Source: CAD feature listing. Evaluate the final solid. Frame: model axes, mm. Face numbers are marked on the shaded views. A direction names the side the tool comes from. Give positions to 0.01 mm unless a question says otherwise; leave off trailing zeros. Loops run counter-clockwise (first coordinate to the right, second up) from the corner with the lowest first, then second, coordinate; pieces in that order, holes last.
from build123d import *

# Parameters (mm, degrees)
SKETCH1_R           = 16
BOSS_EXTRUDE1_DEPTH = 850
SKETCH2_R           = 14.5
CUT_EXTRUDE1_DEPTH  = 848
BOSS_EXTRUDE2_START = -2
SKETCH3_R           = 17
SKETCH3_R_2         = 16
BOSS_EXTRUDE2_DEPTH = 2
FILLET1_R           = 1.5
SKETCH4_R           = 17
SKETCH4_R_2         = 16
BOSS_EXTRUDE3_DEPTH = 2
FILLET2_R           = 1.5


with BuildPart() as part:
    # Sketch1 → Boss-Extrude1 (new body)
    with BuildSketch(Plane(origin=(0, 0, 0), x_dir=(1, 0, 0), z_dir=(0, 1, 0))):
        with Locations(Location((0, 0, 0), (0, 0, 270))):
            Circle(SKETCH1_R)
    extrude(amount=BOSS_EXTRUDE1_DEPTH)

    # Sketch2 → Cut-Extrude1 (cut)
    with BuildSketch(Plane(origin=(0, 850, 0), x_dir=(1, 0, 0), z_dir=(0, 1, 0))):
        with Locations(Location((0, 0, 0), (0, 0, 270))):
            Circle(SKETCH2_R)
    extrude(amount=-CUT_EXTRUDE1_DEPTH, mode=Mode.SUBTRACT)

    # Sketch3 → Boss-Extrude2 (add)
    with BuildSketch(Plane(origin=(0, 800, 0), x_dir=(1, 0, 0), z_dir=(0, 1, 0)).offset(BOSS_EXTRUDE2_START)):
        with Locations(Location((0, 0, 0), (0, 0, 270))):
            Circle(SKETCH3_R)
        with Locations(Location((0, 0, 0), (0, 0, 270))):
            Circle(SKETCH3_R_2, mode=Mode.SUBTRACT)
    extrude(amount=BOSS_EXTRUDE2_DEPTH)

    # Fillet1
    # the kernel refuses this fillet: 1.5 mm, written as the material it takes off along each edge
    with BuildSketch(Plane(origin=(0, 798, 0), x_dir=(0, 0, 1), z_dir=(-1, 0, 0))) as fillet1_piece_1:
        with BuildLine():
            CenterArc((15.5, 1.414213562), FILLET1_R, 289.471220634, 70.528779366)
            Line((17, 1.414213562), (17.03, 1.414213562))
            Line((17.03, 1.414213562), (17.03, 0))
            Line((17.03, 0), (17, -0.03))
            ThreePointArc((17, -0.03), (16.5, -0.03), (16.01, -0.028284271))
            Line((16.01, -0.028284271), (16, 0))
        make_face()
    revolve(axis=Axis((0, 798, 0), (0, 1, 0)), mode=Mode.SUBTRACT)

    # Sketch4 → Boss-Extrude3 (add)
    with BuildSketch(Plane(origin=(0, 640, 0), x_dir=(1, 0, 0), z_dir=(0, 1, 0))):
        with Locations(Location((0, 0, 0), (0, 0, 270))):
            Circle(SKETCH4_R)
        with Locations(Location((0, 0, 0), (0, 0, 270))):
            Circle(SKETCH4_R_2, mode=Mode.SUBTRACT)
    extrude(amount=BOSS_EXTRUDE3_DEPTH)

    # Fillet2
    # the kernel refuses this fillet: 1.5 mm, written as the material it takes off along each edge
    with BuildSketch(Plane(origin=(0, 642, 0), x_dir=(0, 0, 1), z_dir=(-1, 0, 0))) as fillet2_piece_1:
        with BuildLine():
            CenterArc((15.5, -1.414213562), FILLET2_R, 0, 70.528779366)
            Line((16, 0), (16.01, 0.028284271))
            ThreePointArc((16.01, 0.028284271), (16.5, 0.03), (17, 0.03))
            Line((17, 0.03), (17.03, 0))
            Line((17.03, 0), (17.03, -1.414213562))
            Line((17.03, -1.414213562), (17, -1.414213562))
        make_face()
    revolve(axis=Axis((0, 642, 0), (0, 1, 0)), mode=Mode.SUBTRACT)


solid = part.part
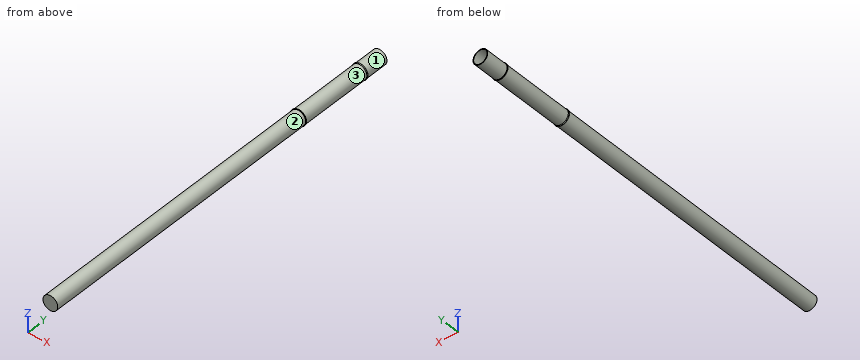
1) Cut plane B-B (y = 126). Return loops of the section in (x, z).
Checks:
outline: circle Ø32 at (0, 0); hole circle Ø29 at (0, 0)
2) Contact query for flat-ended pins moving along their axis: P1, Ø17, axis at x = -3.5, z = 0, coming from the -Y side; P2, Ø5, axis at x = 13.5, y = 373, coming from the +Z side; P3, Ø10, axis at y = 727, z = 12, coming from the +X side; P4, Ø6, axis at x = 4.5, y = 264, coming from the -Z side. Output: stop coordinate, or through.
Checks:
P1: stops at y = 0
P2: stops at z = 11.62
P3: stops at x = 14.39
P4: stops at z = -15.93
3) Cut plane A-A (z = 0). Return loops of the section in (x, y).
Checks:
outline: (-17, 640) - (-16, 640) - (-16, 0) - (16, 0) - (16, 640) - (17, 640) - (17, 640.59) arc R1.5 ccw to (16, 642) - (16, 798) arc R1.5 ccw to (17, 799.41) - (17, 800) - (16, 800) - (16, 850) - (14.5, 850) - (14.5, 2) - (-14.5, 2) - (-14.5, 850) - (-16, 850) - (-16, 800) - (-17, 800) - (-17, 799.41) arc R1.5 ccw to (-16, 798) - (-16, 642) arc R1.5 ccw to (-17, 640.59) - close
4) Ray query, probe 1 along X at (y, z) = (201, 0); probe 2 along Z at (x, y) = (1, 394); probe 3 along X at (y, z) = (269, 2). Return the intervals inside material, ascending.
Checks:
probe 1: x = -16 to -14.5, 14.5 to 16
probe 2: z = -15.97 to -14.47, 14.47 to 15.97
probe 3: x = -15.87 to -14.36, 14.36 to 15.87
5) Reachability of the marked faces 1, 2 and 3 from +Z, -Z, +X, -X, +Y, -Y: full face, straight path, thin tool, end or side. Return the list, or none.
Checks:
face 1: +Y
face 2: -Y
face 3: none
